from build123d import *

# Parameters (mm, degrees)
SKETCH1_R                = 3.05
BOSS_EXTRUDE1_DEPTH      = 100
BOSS_EXTRUDE2_DEPTH      = 28.5
BOSS_EXTRUDE2_DEPTH_BACK = 28.5
SKETCH3_R                = 2.5
SKETCH3_R_2              = 1.5
BOSS_EXTRUDE3_DEPTH      = 1.5
CHAMFER1_SIZE            = 0.5
SKETCH4_R                = 4.3
SKETCH4_R_2              = 2.3
BOSS_EXTRUDE4_DEPTH      = 3
CUT_EXTRUDE1_START       = -3
SKETCH4_2_R              = 2.3
CUT_EXTRUDE1_DEPTH       = 3


with BuildPart() as part:
    # Sketch1 → Boss-Extrude1 (new, symmetric)
    with BuildSketch(Plane(origin=(0, 0, 0), x_dir=(1, 0, 0), z_dir=(0, 1, 0))):
        with BuildLine():
            Line((-28.5, 5.55), (28.5, 5.55))
            ThreePointArc((28.5, 5.55), (34.05, 0), (28.5, -5.55))
            Line((28.5, -5.55), (-28.5, -5.55))
            ThreePointArc((-28.5, -5.55), (-34.05, 0), (-28.5, 5.55))
        make_face()
        with Locations(Location((-28.5, 0, 0), (0, 0, 270))):
            Circle(SKETCH1_R, mode=Mode.SUBTRACT)
        with Locations(Location((28.5, 0, 0), (0, 0, 270))):
            Circle(SKETCH1_R, mode=Mode.SUBTRACT)
    extrude(amount=BOSS_EXTRUDE1_DEPTH, both=True)

    # Sketch2 → Boss-Extrude2 (add, two sides: drawn at the far end of the back side and taken through both)
    with BuildSketch(Plane(origin=(0, 0, 0), x_dir=(0, 0, -1), z_dir=(1, 0, 0)).offset(-BOSS_EXTRUDE2_DEPTH_BACK)):
        Polygon((5.55, 36.664900987), (5.55, -0.532059786), (7.05, -0.532059786), (14.82084997, 36.664900987), align=None)
    extrude(amount=BOSS_EXTRUDE2_DEPTH + BOSS_EXTRUDE2_DEPTH_BACK)

    # Sketch3 → Boss-Extrude3 (add)
    # profile 1 of 4: a face of its own
    with BuildSketch(Plane(origin=(0, -1.433480354, -6.861683432), x_dir=(-1, 0, 0), z_dir=(0, -0.20449605184178382, -0.9788673887616864))):
        with Locations(Location((-14, 33.920881193, 0), (0, 0, 270))):
            Circle(SKETCH3_R)
        with Locations(Location((-14, 33.920881193, 0), (0, 0, 270))):
            Circle(SKETCH3_R_2, mode=Mode.SUBTRACT)
    # profile 2 of 4: a face of its own
    with BuildSketch(Plane(origin=(0, -1.433480354, -6.861683432), x_dir=(-1, 0, 0), z_dir=(0, -0.20449605184178382, -0.9788673887616864))):
        with Locations(Location((14, 33.920881193, 0), (0, 0, 270))):
            Circle(SKETCH3_R)
        with Locations(Location((14, 33.920881193, 0), (0, 0, 270))):
            Circle(SKETCH3_R_2, mode=Mode.SUBTRACT)
    # profile 3 of 4: a face of its own
    with BuildSketch(Plane(origin=(0, -1.433480354, -6.861683432), x_dir=(-1, 0, 0), z_dir=(0, -0.20449605184178382, -0.9788673887616864))):
        with Locations(Location((14, 5.920881193, 0), (0, 0, 270))):
            Circle(SKETCH3_R)
        with Locations(Location((14, 5.920881193, 0), (0, 0, 270))):
            Circle(SKETCH3_R_2, mode=Mode.SUBTRACT)
    # profile 4 of 4: a face of its own
    with BuildSketch(Plane(origin=(0, -1.433480354, -6.861683432), x_dir=(-1, 0, 0), z_dir=(0, -0.20449605184178382, -0.9788673887616864))):
        with Locations(Location((-14, 5.920881193, 0), (0, 0, 270))):
            Circle(SKETCH3_R)
        with Locations(Location((-14, 5.920881193, 0), (0, 0, 270))):
            Circle(SKETCH3_R_2, mode=Mode.SUBTRACT)
    extrude(amount=BOSS_EXTRUDE3_DEPTH)

    # Chamfer1
    chamfer1_edges = [part.edges().sort_by_distance(p)[0] for p in [
        (14, 33.910988438, -15.777910924),
        (-14, 33.910988438, -15.777910924),
        (-14, 6.502701552, -10.052021472),
        (14, 6.502701552, -10.052021472),
    ]]
    chamfer(chamfer1_edges, length=CHAMFER1_SIZE)

    # Sketch4 → Boss-Extrude4 (add)
    # profile 1 of 4: a face of its own
    with BuildSketch(Plane.XY.offset(5.55)):
        with Locations(Location((-22, 77, 0), (0, 0, 180))):
            Circle(SKETCH4_R)
        with Locations((-22, 77)):
            Circle(SKETCH4_R_2, mode=Mode.SUBTRACT)
    # profile 2 of 4: a face of its own
    with BuildSketch(Plane.XY.offset(5.55)):
        with Locations(Location((22, 77, 0), (0, 0, 180))):
            Circle(SKETCH4_R)
        with Locations((22, 77)):
            Circle(SKETCH4_R_2, mode=Mode.SUBTRACT)
    # profile 3 of 4: a face of its own
    with BuildSketch(Plane.XY.offset(5.55)):
        with Locations(Location((-22, -11, 0), (0, 0, 180))):
            Circle(SKETCH4_R)
        with Locations((-22, -11)):
            Circle(SKETCH4_R_2, mode=Mode.SUBTRACT)
    # profile 4 of 4: a face of its own
    with BuildSketch(Plane.XY.offset(5.55)):
        with Locations(Location((22, -11, 0), (0, 0, 180))):
            Circle(SKETCH4_R)
        with Locations((22, -11)):
            Circle(SKETCH4_R_2, mode=Mode.SUBTRACT)
    extrude(amount=BOSS_EXTRUDE4_DEPTH)

    # Sketch4<2> → Cut-Extrude1 (cut)
    with BuildSketch(Plane.XY.offset(5.55).offset(CUT_EXTRUDE1_START)):
        with Locations((22, 77)):
            Circle(SKETCH4_2_R)
        with Locations((-22, 77)):
            Circle(SKETCH4_2_R)
        with Locations((22, -11)):
            Circle(SKETCH4_2_R)
        with Locations((-22, -11)):
            Circle(SKETCH4_2_R)
    extrude(amount=CUT_EXTRUDE1_DEPTH, mode=Mode.SUBTRACT)


solid = part.part
Geometry: final body of the model. Coordinates: model frame, mm. A direction names the side the tool comes from. Give positions to 0.01 mm unless a question says otherwise; leave off trailing zeros. Write each loop counter-clockwise with the first axis right and the second up, starting at its lowest first coordinate (ties: lowest second). Pieces come first, ordered by that corner, then holes. Notation, with made-up numbers: M 56,54.5 L 71,54.5 A20 cw 71,61.5 Z; hole C 42.5,-17.75 d11. An arc over 180 degrees is marked long. Answer in a Markdown table with one row per item. Add a question column.
(1) Section D-D on y = -11. Return loops of the section in (x, z).
(2) Section B-B on y = -86.5. Return loops of the section in (x, z).
(3) Section C-C on x = 22. Return loops of the section in (y, z).
(4) First-contact query: pin 1 (6 mm diameter, centred on x = 22, y = -11, fed in from -Z); pin 2 (1 mm diameter, centred on x = 27, y = 30, fed in from -Z); pin 3 (1.5 mm diameter, centred on x = -11, z = -10.5, fed in from +Y). Flat tips, straight axial feed; report the tip coordinate or a pass-through.
(5) Reachability of faces 4 (the cylindrical face through (-21.44, 72.737, 7.029)), 5 (the cylindrical face through (16.44, 4.79, -8.67)) from +Z, -Z, +X, -X, +Y, -Y: full face, straight path, thin tool, end or side. Return the list, or none.
(6) Section A-A on z = 0. Return loops of the section in (x, y).
(7) Mould query, pull axis X, two halves, no side actions, for faces 1 (the cylindrical face through (-12.48, 33.61, -14.69)), 2 (the flat face through (-28.5, 22, -9)), 3 (the flat face through (0, 100, 0)). Classes: +X half, -X half, draft (parallel to the pull), parting line (faces both ways), or undercut.
(8) Ray query, line 1 (X direction, y = 60, z = 0); line 2 (Y direction, x = -22, z = 4.5); line 3 (Y direction, x = 22, z = 6.25). Return the intervals inside material, ascending.
Result set:
| question | item | result |
|---|---|---|
| 1 | outline | M -28.5,-5.55 L 28.5,-5.55 A5.55 ccw 28.5,5.55 L 26.3,5.55 L 26.3,8.55 L 24.3,8.55 L 24.3,2.55 L 19.7,2.55 L 19.7,8.55 L 17.7,8.55 L 17.7,5.55 L -17.7,5.55 L -17.7,8.55 L -19.7,8.55 L -19.7,2.55 L -24.3,2.55 L -24.3,8.55 L -26.3,8.55 L -26.3,5.55 L -28.5,5.55 A5.55 ccw Z; hole C -28.5,0 d6.1; hole C 28.5,0 d6.1 |
| 2 | outline | M -28.5,-5.55 L 28.5,-5.55 A5.55 ccw 28.5,5.55 L -28.5,5.55 A5.55 ccw Z; hole C -28.5,0 d6.1; hole C 28.5,0 d6.1 |
| 3 | outline | M -100,-5.55 L -0.53,-5.55 L -0.53,-7.05 L 36.66,-14.82 L 36.66,-5.55 L 100,-5.55 L 100,5.55 L 81.3,5.55 L 81.3,8.55 L 79.3,8.55 L 79.3,2.55 L 74.7,2.55 L 74.7,8.55 L 72.7,8.55 L 72.7,5.55 L -6.7,5.55 L -6.7,8.55 L -8.7,8.55 L -8.7,2.55 L -13.3,2.55 L -13.3,8.55 L -15.3,8.55 L -15.3,5.55 L -100,5.55 Z |
| 4 | pin 1 | stops at z = -5.55 |
| 4 | pin 2 | stops at z = -13.53 |
| 4 | pin 3 | stops at y = 36.66 |
| 5 | face 4 | +Z |
| 5 | face 5 | none |
| 6 | outline | M -34.05,-100 L -31.55,-100 L -31.55,100 L -34.05,100 Z; M -25.45,-100 L 25.45,-100 L 25.45,100 L -25.45,100 Z; M 31.55,-100 L 34.05,-100 L 34.05,100 L 31.55,100 Z |
| 7 | face 1 | undercut |
| 7 | face 2 | -X half |
| 7 | face 3 | draft |
| 8 | line 1 | x = -34.05 to -31.55, -25.45 to 25.45, 31.55 to 34.05 |
| 8 | line 2 | y = -100 to -13.3, -8.7 to 74.7, 79.3 to 100 |
| 8 | line 3 | y = -15.3 to -13.3, -8.7 to -6.7, 72.7 to 74.7, 79.3 to 81.3 |
